Part model, mm, in its own coordinate system. A direction names the side the tool comes from. Give positions to 0.01 mm unless a question says otherwise; leave off trailing zeros. Order: outer loops, then holes, each group sorted by start corner. A loop starts at its lowest first (then second) coordinate and runs counter-clockwise, first axis right, second up. Notation, with made-up numbers: (-23, -1.5) - (7, -1.5) arc R33 ccw to (7, 27.5) - close; hole circle Ø2 at (23, 32.5). An arc over 180 degrees is marked (long way). One line per item, written item: value.
```python
from build123d import *

# Parameters (mm, degrees)
SKETCH_W        = 69
SKETCH_H        = 69.5
SKETCH_R        = 2.55
PAD_DEPTH       = 4.5
SKETCH001_W     = 69
SKETCH001_H     = 69.5
SKETCH001_W_2   = 65
SKETCH001_H_2   = 65.5
PAD001_DEPTH    = 40
POCKET_DEPTH    = 69.001
SKETCH003_R     = 4.55
POCKET001_DEPTH = 3
FILLET_R        = 1.8


with BuildPart() as part:
    # Sketch → Pad (new body)
    with BuildSketch(Plane.XZ):
        Rectangle(SKETCH_W, SKETCH_H)
        with Locations((-24, 24)):
            Circle(SKETCH_R, mode=Mode.SUBTRACT)
        with Locations((24, 24)):
            Circle(SKETCH_R, mode=Mode.SUBTRACT)
        with Locations((-24, -24)):
            Circle(SKETCH_R, mode=Mode.SUBTRACT)
        with Locations((24, -24)):
            Circle(SKETCH_R, mode=Mode.SUBTRACT)
        with BuildLine():
            Line((-18, 30.75), (18, 30.75))
            Line((18, 30.75), (18, 24))
            ThreePointArc((18, 24), (19.757359, 19.757359), (24, 18))
            Line((24, 18), (30.5, 18))
            Line((30.5, 18), (30.5, -18))
            Line((23.999998, -18), (30.5, -18))
            ThreePointArc((23.999998, -18), (19.757359, -19.75736), (18, -24))
            Line((18, -30.75), (18, -24))
            Line((18, -30.75), (-18, -30.75))
            Line((-18, -24), (-18, -30.75))
            ThreePointArc((-18, -24), (-19.757359, -19.757359), (-24, -18))
            Line((-30.5, -18), (-24, -18))
            Line((-30.5, -18), (-30.5, 18))
            Line((-30.5, 18), (-24, 18))
            ThreePointArc((-24, 18), (-19.757359, 19.757359), (-18, 24))
            Line((-18, 30.75), (-18, 24))
        make_face(mode=Mode.SUBTRACT)
    extrude(amount=PAD_DEPTH)

    # Sketch001 → Pad001 (join)
    with BuildSketch(Plane.XZ):
        Rectangle(SKETCH001_W, SKETCH001_H)
        Rectangle(SKETCH001_W_2, SKETCH001_H_2, mode=Mode.SUBTRACT)
    extrude(amount=PAD001_DEPTH)

    # Sketch002 (on Face7 of Pad001) → Pocket (cut, through all)
    with BuildSketch(Plane(origin=(-34.5, 0, 0), x_dir=(0, 0, -1), z_dir=(-1, 0, 0))):
        Polygon((-34.75, 14.5), (24.75, 40), (-34.75, 40), align=None)
    extrude(amount=-POCKET_DEPTH, mode=Mode.SUBTRACT)

    # Sketch003 (on Face37 of Pocket) → Pocket001 (cut)
    with BuildSketch(Plane.XZ.offset(4.5)):
        with Locations((-24, 24)):
            Circle(SKETCH003_R)
        with Locations((24, 24)):
            Circle(SKETCH003_R)
        with Locations((-24, -24)):
            Circle(SKETCH003_R)
        with Locations((24, -24)):
            Circle(SKETCH003_R)
    extrude(amount=-POCKET001_DEPTH, mode=Mode.SUBTRACT)

    # Fillet
    fillet_edges = [part.edges().sort_by_distance(p)[0] for p in [
        (-34.5, -9.5, 34.75),
        (-34.5, -2.25, 34.75),
        (-34.5, -2.25, -34.75),
        (-34.5, -22.25, -34.75),
        (34.5, -22.25, -34.75),
        (34.5, -2.25, -34.75),
        (34.5, -9.5, 34.75),
        (34.5, -2.25, 34.75),
    ]]
    fillet(fillet_edges, radius=FILLET_R)


solid = part.part
```
1) Mould opens along X. For faces 3 (the flat face through (-21, 0, 23)), 4 (the flat face through (-34.5, -15, -8)), 5 (the cylindrical face through (19.711, -2.218, 19.804)) say: released by +X, released by -X, zero draft, split by the parting line, or undercut.
Outcome:
face 3: zero draft
face 4: released by -X
face 5: undercut
2) Cut at A-A, the plane z = -12.5. Give the cut face in (x, y).
Outcome:
outline: (-34.5, -34.75) - (-32.5, -34.75) - (-32.5, -4.5) - (-30.5, -4.5) - (-30.5, 0) - (-34.5, 0) - close; (30.5, -4.5) - (32.5, -4.5) - (32.5, -34.75) - (34.5, -34.75) - (34.5, 0) - (30.5, 0) - close
3) Drill centre lines: line 1 along Z through (x, y) = (24, -3); line 2 along Z through (x, y) = (24, -0.6); line 3 along X through (y, z) = (-0.55, -24). Where is each one in solid material? Low to high. Write a range as from..to.
Outcome:
line 1: z = -34.75..-28.55, -19.45..-18, 18..19.45, 28.55..34.75
line 2: z = -34.75..-26.55, -21.45..-18, 18..21.45, 26.55..34.75
line 3: x = -34.5..-26.55, -21.45..-18, 18..21.45, 26.55..34.5
4) Which spindle directions (+Z, -Z, +X, -X, +Y, -Y) get a long thin tool onto all of the face, cutting with end or side? Do faces 1 (the flat face through (-22, -4.5, -19)), 2 (the flat face through (27, -2, 18)). Say none if no direction does.
Outcome:
face 1: -Y
face 2: +Y, -Y
5) Cut at D-D, the plane z = 25. Give the cut face in (x, y).
Outcome:
outline: (-34.5, -18.68) - (-32.5, -18.68) - (-32.5, -4.5) - (-28.44, -4.5) - (-28.44, -1.5) - (-26.35, -1.5) - (-26.35, 0) - (-34.5, 0) - close; (-21.65, -1.5) - (-19.56, -1.5) - (-19.56, -4.5) - (-18, -4.5) - (-18, 0) - (-21.65, 0) - close; (18, -4.5) - (19.56, -4.5) - (19.56, -1.5) - (21.65, -1.5) - (21.65, 0) - (18, 0) - close; (26.35, -1.5) - (28.44, -1.5) - (28.44, -4.5) - (32.5, -4.5) - (32.5, -18.68) - (34.5, -18.68) - (34.5, 0) - (26.35, 0) - close
6) Cut at C-C, the plane y = -8.5. Give the cut face in (x, z).
Outcome:
outline: (-34.5, -32.95) arc R1.8 ccw to (-32.7, -34.75) - (32.7, -34.75) arc R1.8 ccw to (34.5, -32.95) - (34.5, 32.95) arc R1.8 ccw to (32.7, 34.75) - (-32.7, 34.75) arc R1.8 ccw to (-34.5, 32.95) - close; hole (-32.5, -32.75) - (32.5, -32.75) - (32.5, 32.75) - (-32.5, 32.75) - close
7) Pin check, flat tips, straight feed: pin 1 (8 mm diameter, centred on x = -24, z = 24, fed in from -Y); pin 2 (7.5 mm diameter, centred on x = -22, z = 26, fed in from -Y); pin 3 (1.5 mm diameter, centred on x = -6.5, y = -30.5, fed in from +Z). Stop position of each tip, or through.
Outcome:
pin 1: stops at y = -1.5
pin 2: stops at y = -4.5
pin 3: stops at z = -32.75
8) Cut at B-B, the plane x = 7. Give the cut face in (y, z), then the cut area to 3 significant figures.
Outcome:
outline: (-40, -34.75) - (0, -34.75) - (0, -30.75) - (-4.5, -30.75) - (-4.5, -32.75) - (-40, -32.75) - close; (-15.36, 32.75) - (-4.5, 32.75) - (-4.5, 30.75) - (0, 30.75) - (0, 34.75) - (-14.5, 34.75) - close
area: 128 mm^2
